For this review, use the dimensioned drawing (mm, ordinates from the lowest corner) and the shaded views. A direction names the side the tool comes from. Coordinates: 2 decimals unless noted, no trailing zeros. Write each loop counter-clockwise with the first axis right and the second up, starting at its lowest first coordinate (ties: lowest second). Pieces come first, ordered by that corner, then holes. Notation, with made-up numbers: M 6,20.5 L 43,20.5 A23 ccw 43,45.5 Z; hole C -5.75,-4.5 d11. An arc over 180 degrees is marked long. Return JSON: item names as keys, results as strings. Group by question number.
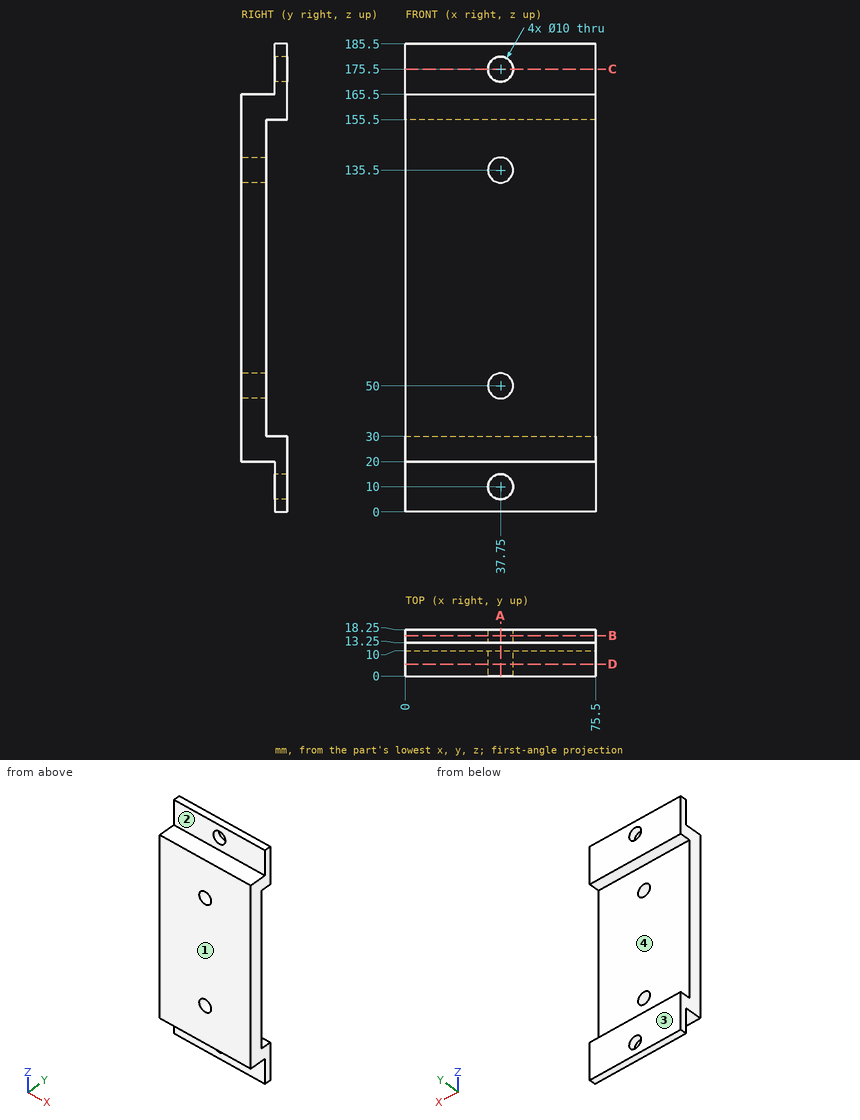
Item 1: The part is to be moulded in two halves that separate along Z. For the marked faces 3 and 4, say which applies: pulls with the +Z half, pulls with the -Z half, needs draft (parallel to the pull), parting line crosses it, or undercut.
Item 2: For line 1 (Z direction, x = 37.75, y = 2.75); line 2 (Z direction, x = 37.75, y = 16.3); line 3 (Z direction, x = 72.5, y = 17.25), list the stretches that pass through material, from the lowest coordinate up.
Item 3: Machinability: for the marked faces 1 and 2, which of the approach directions +Z, -Z, +X, -X, +Y, -Y give a long, thin tool a straight path to every point of the face, cutting with its end or side? Answer none if there is none.
Item 4: Add section B-B (y = 16). Write out the cut boundary in (x, z), plus the area to 3 significant figures.
Item 5: Add section D-D (y = 4.75). Write out the cut boundary in (x, z), plus the area to 3 significant figures.
Item 6: Add section C-C (z = 175.5). Write out the cut boundary in (x, y).
Item 7: For pin 1 (6.5 mm diameter, centred on x = 56, y = 8.5, fed in from -Z); pin 2 (13 mm diameter, centred on x = 37.75, z = 135.5, fed in from +Y); pin 3 (4 mm diameter, centred on x = 24, y = 9.5, fed in from +Z); pin 4 (9 mm diameter, centred on x = 37.75, z = 10, fed in from -Y), all flat-tipped, find the tip position at first contact; note any pin that passes through.
Item 8: Add section A-A (x = 37.75). Write out the cut boundary in (y, z), plus the area to 3 significant figures.
Geometry check:
{
 "1": {"face 3": "needs draft", "face 4": "undercut"},
 "2": {"line 1": "20 to 45, 55 to 130.5, 140.5 to 165.5", "line 2": "0 to 5, 15 to 30, 155.5 to 170.5, 180.5 to 185.5", "line 3": "0 to 30, 155.5 to 185.5"},
 "3": {"face 1": "+Z, -Z, +X, -X, -Y", "face 2": "+Z, +X, -X, -Y"},
 "4": {"outline": "M 0,0 L 75.5,0 L 75.5,30 L 0,30 Z; M 0,155.5 L 75.5,155.5 L 75.5,185.5 L 0,185.5 Z; hole C 37.75,10 d10; hole C 37.75,175.5 d10", "area": "4,370 mm^2"},
 "5": {"outline": "M 0,20 L 75.5,20 L 75.5,165.5 L 0,165.5 Z; hole C 37.75,50 d10; hole C 37.75,135.5 d10", "area": "10,800 mm^2"},
 "6": {"outline": "M 0,13.25 L 32.75,13.25 L 32.75,18.25 L 0,18.25 Z; M 42.75,13.25 L 75.5,13.25 L 75.5,18.25 L 42.75,18.25 Z"},
 "7": {"pin 1": "z = 20", "pin 2": "y = 10", "pin 3": "z = 165.5", "pin 4": "through"},
 "8": {"outline": "M 0,20 L 13.25,20 L 13.25,15 L 18.25,15 L 18.25,30 L 10,30 L 10,45 L 0,45 Z; M 0,55 L 10,55 L 10,130.5 L 0,130.5 Z; M 0,140.5 L 10,140.5 L 10,155.5 L 18.25,155.5 L 18.25,170.5 L 13.25,170.5 L 13.25,165.5 L 0,165.5 Z; M 13.25,0 L 18.25,0 L 18.25,5 L 13.25,5 Z; M 13.25,180.5 L 18.25,180.5 L 18.25,185.5 L 13.25,185.5 Z", "area": "1,520 mm^2"}
}
